Part model, mm, in its own coordinate system. A direction names the side the tool comes from. Coordinates: 2 decimals unless noted, no trailing zeros. Write each loop counter-clockwise with the first axis right and the second up, starting at its lowest first coordinate (ties: lowest second). Pieces come first, ordered by that corner, then holes. Notation, with made-up numbers: (-10, 24) - (20, 24) arc R13 ccw to (20, 32) - close; hole circle Ø5 at (-22, 43). An arc over 180 degrees is marked (long way). Write each question's results on one line, items separated by ' | '.
Autodesk Inventor part; units mm, degrees
ref_plane "YZ Plane" through (0, 0, 0) normal (1, 0, 0) x (0, 1, 0)
ref_plane "XZ Plane" through (0, 0, 0) normal (0, 1, 0) x (-1, 0, 0)
ref_plane "XY Plane" through (0, 0, 0) normal (0, 0, 1) x (1, 0, 0)
sketch "Sketch1" plane through (0, 0, 0) normal (0, 0, 1) x (1, 0, 0)
  circle A0 centre (0, 0) radius 6
  circle A1 centre (0, 0) radius 3
  dimension "d0" = 12
  dimension "d1" = 6
extrude "Extrusion1" add sketch "Sketch1" along normal blind 15.5
sketch "Sketch2" plane through (0, 0, 15.5) normal (0, 0, 1) x (1, 0, 0)
  line L0 (-4, 6) -> (4, 6)
  line L1 (4, 6) -> (4, -6)
  line L2 (4, -6) -> (-4, -6)
  line L3 (-4, -6) -> (-4, 6)
  circle A0 centre (0, 0) radius 6 construction
  point P0 (0, 6)
  point P1 (4, 0)
  point P2 (0, -6)
  dimension "d4" = 8
extrude "Extrusion2" cut sketch "Sketch2" against normal blind 7.75
sketch "Sketch3" plane through (-4, -4.4721, 15.5) normal (1, 0, 0) x (0, 0, -1)
  arc A0 (2, 8.9443) -> (0, 6.9443) centre (2, 6.9443) ccw
  line L0 (0, 0) -> (7.75, 0)
  line L1 (7.75, 0) -> (7.75, 0)
  line L2 (7.75, 0) -> (0, 0)
  line L3 (0, 8.9443) -> (0, 0)
  line L4 (0, 8.9443) -> (7.75, 8.9443)
  line L5 (7.75, 8.9443) -> (7.75, 8.9443)
  line L6 (7.75, 8.9443) -> (0, 8.9443)
  line L7 (0, 0) -> (0, 8.9443)
  line L8 (15.5, -1.5279) -> (15.5, 10.4721)
  line L9 (0, 8.9443) -> (0, 0)
  arc A1 (0, 2) -> (2, 0) centre (2, 2) ccw
  line L10 (0, 2) -> (0, 0)
  line L11 (2, 0) -> (0, 0)
  line L12 (0, 6.9443) -> (0, 8.9443)
  line L13 (2, 8.9443) -> (0, 8.9443)
  point P0 (15.5, 4.4721)
  dimension "d7" = 2
  dimension "d8" = 2
extrude "Extrusion3" cut sketch "Sketch3" along normal through all both and the other way through all
sketch "Sketch4" plane through (-4, -4.4721, 7.75) normal (1, 0, 0) x (0, 0, -1)
  circle A0 centre (-5.75, 4.4721) radius 1.25
  line L0 (-7.75, 6.9443) -> (-7.75, 2)
  point P0 (7.75, 4.4721)
  point P1 (-7.75, 4.4721)
  dimension "d11" = 2.5
  dimension "d12" = 2
extrude "Extrusion4" cut sketch "Sketch4" along normal through all both and the other way through all
sketch "Sketch5" plane through (0, 0, 7.75) normal (0, 0, 1) x (1, 0, 0)
  line L0 (-6, 3) -> (6, 3)
  line L1 (6, 3) -> (6, -3)
  line L2 (6, -3) -> (-6, -3)
  line L3 (-6, -3) -> (-6, 3)
  arc A0 (-5.467, 2.4721) -> (-5.467, -2.4721) centre (0, 0) ccw
  arc A1 (5.467, -2.4721) -> (5.467, 2.4721) centre (0, 0) ccw
  line L4 (-12.5137, 9.699) -> (15.0071, 9.699)
  line L5 (15.0071, 9.699) -> (15.0071, -9.2746)
  line L6 (15.0071, -9.2746) -> (-12.5137, -9.2746)
  line L7 (-12.5137, -9.2746) -> (-12.5137, 9.699)
  point P0 (0, 3)
  point P1 (-6, 0)
  dimension "d15" = 6
extrude "Extrusion5" cut sketch "Sketch5" along normal through all
fillet "Fillet1" radius 2 4 edges at (-4.5981, 3, 15.4291) (-4.5981, -3, 15.4291) (4.5981, 3, 15.4291) (4.5981, -3, 15.4291)
properties part number "P1" material "Steel"
(1) Saw through at A-A on y = 0. Write the cut outline in (x, z).
Return value:
outline: (-6, 0) - (-3, 0) - (-3, 7.75) - (-4, 7.75) - (-4, 12.25) - (-6, 12.25) - close; (-6, 14.75) - (-4, 14.75) - (-4, 15.5) - (-6, 15.5) - close; (3, 0) - (6, 0) - (6, 12.25) - (4, 12.25) - (4, 7.75) - (3, 7.75) - close; (4, 14.75) - (6, 14.75) - (6, 15.5) - (4, 15.5) - close
(2) Wall check: line 1 (X direction, y = 0, z = 6); line 2 (Y direction, x = 4.9, z = 13.5); line 3 (Z direction, x = 5.25, y = 0). Give the ranges that are in metal, low to high. Write a range as from..to.
Return value:
line 1: x = -6..-3, 3..6 | line 2: y = -3..-1.25, 1.25..3 | line 3: z = 0..12.25, 14.75..15.5
(3) 3-axis set-ups, long thin cutter, end or side, ignore diameter. For faces 4 (the cylindrical face through (-4.986, -0.479, 12.345)), 5 (the flat face through (-4, 0, 12)), 6 (the flat face through (5, -3, 11)), 7 (the flat face through (5, 3, 11)): which of +Z, -Z, +X, -X, +Y, -Y reach the whole face in a straight line?
Return value:
face 4: +X, -X | face 5: +Z, +Y, -Y | face 6: +Z, +X, -X, -Y | face 7: +Z, +X, -X, +Y
(4) Two-plate mould, pull along X, no slides. Class faces 1 (the cylindrical face through (4.986, 0.479, 12.345)), 2 (the flat face through (-1, 3, 7.75)), 3 (the cylindrical face through (5.54, 2.3, 5.92)): released by +X, released by -X, zero draft, split by the parting line, or undercut.
Return value:
face 1: zero draft | face 2: undercut | face 3: split by the parting line
(5) Saw through at C-C on x = 4.75. Write the cut outline in (y, z), then the cut area to 3 significant figures.
Return value:
outline: (-3.67, 0) - (3.67, 0) - (3.67, 7.75) - (3, 7.75) - (3, 13.5) arc R2 ccw to (1, 15.5) - (-1, 15.5) arc R2 ccw to (-3, 13.5) - (-3, 7.75) - (-3.67, 7.75) - close; hole circle Ø2.5 at (0, 13.5) | area: 96.7 mm^2
(6) Saw through at B-B on x = 0. Write the cut outline in (y, z).
Return value:
outline: (-6, 0) - (-3, 0) - (-3, 7.75) - (-6, 7.75) - close; (3, 0) - (6, 0) - (6, 7.75) - (3, 7.75) - close
(7) Flat gauge pins, fed straight in: P1, Ø6, axis at y = 4.5, z = 14, coming from the -X side; P2, Ø3, axis at x = -0.5, y = 3, coming from the +Z side; P3, Ø1, axis at x = -4.5, z = 11.5, coming from the +Y side. Where does each tip first touch, or does it go through?
Return value:
P1: stops at x = -5.81 | P2: stops at z = 7.75 | P3: stops at y = 3
(8) Saw through at D-D on z = 12.5. Write the cut outline in (x, y).
Return value:
outline: (-5.95, -0.75) arc R6 ccw to (-5.2, -3) - (-4, -3) - (-4, -0.75) - close; (-5.95, 0.75) - (-4, 0.75) - (-4, 3) - (-5.2, 3) arc R6 ccw to start; (4, -3) - (5.2, -3) arc R6 ccw to (5.95, -0.75) - (4, -0.75) - close; (4, 0.75) - (5.95, 0.75) arc R6 ccw to (5.2, 3) - (4, 3) - close
